Design review of the part built by this model. Coordinates are the model's own, in mm. A direction names the side the tool comes from. Give positions to 0.01 mm unless a question says otherwise; leave off trailing zeros. Order: outer loops, then holes, each group sorted by start corner. A loop starts at its lowest first (then second) coordinate and runs counter-clockwise, first axis right, second up. Notation, with made-up numbers: (63, 51.5) -> (92, 51.5) arc R29 cw to (92, 81.5) -> close; hole circle Ø6 at (30, -40). An arc over 180 degrees is marked (long way). One line per item, written item: value.
from build123d import *

# Parameters (mm, degrees)
SKETCH1_W           = 85
SKETCH1_H           = 115
SKETCH1_R           = 4.25
SKETCH1_R_2         = 8.5
SKETCH1_R_3         = 6.25
SKETCH1_R_4         = 2.5
SKETCH1_W_2         = 28
SKETCH1_H_2         = 17
BOSS_EXTRUDE1_DEPTH = 3
SKETCH2_W           = 88.917707464
SKETCH2_H           = 119.141928202
SKETCH2_W_2         = 85
SKETCH2_H_2         = 115
BOSS_EXTRUDE2_DEPTH = 50
SKETCH3_R           = 6
BOSS_EXTRUDE3_DEPTH = 50
SKETCH5_R           = 1.6
CUT_EXTRUDE1_DEPTH  = 30


with BuildPart() as part:
    # Sketch1 → Boss-Extrude1 (new body)
    with BuildSketch(Plane(origin=(0, 0, 0), x_dir=(1, 0, 0), z_dir=(0, 1, 0))):
        Rectangle(SKETCH1_W, SKETCH1_H)
        with Locations((-7.5, 47.5)):
            Circle(SKETCH1_R, mode=Mode.SUBTRACT)
        with Locations((-21, 21.25)):
            Circle(SKETCH1_R_2, mode=Mode.SUBTRACT)
        with Locations((6, 21.25)):
            Circle(SKETCH1_R_2, mode=Mode.SUBTRACT)
        with Locations((24.83030278, -21)):
            Circle(SKETCH1_R_3, mode=Mode.SUBTRACT)
        with Locations((24.83030278, -40)):
            Circle(SKETCH1_R_4, mode=Mode.SUBTRACT)
        with Locations((-7.5, -4.5)):
            Rectangle(SKETCH1_W_2, SKETCH1_H_2, mode=Mode.SUBTRACT)
    extrude(amount=BOSS_EXTRUDE1_DEPTH)

    # Sketch2 → Boss-Extrude2 (add)
    with BuildSketch(Plane(origin=(0, 3, 0), x_dir=(1, 0, 0), z_dir=(0, 1, 0))):
        Rectangle(SKETCH2_W, SKETCH2_H)
        Rectangle(SKETCH2_W_2, SKETCH2_H_2, mode=Mode.SUBTRACT)
    extrude(amount=-BOSS_EXTRUDE2_DEPTH)

    # Sketch3 → Boss-Extrude3 (add)
    with BuildSketch(Plane(origin=(0, 3, 0), x_dir=(1, 0, 0), z_dir=(0, 1, 0))):
        with Locations((44.458853732, 59.570964101)):
            Circle(SKETCH3_R)
        with Locations((-44.458853732, 59.570964101)):
            Circle(SKETCH3_R)
        with Locations((44.458853732, -59.570964101)):
            Circle(SKETCH3_R)
        with Locations((-44.458853732, -59.570964101)):
            Circle(SKETCH3_R)
    extrude(amount=-BOSS_EXTRUDE3_DEPTH)

    # Sketch5 → Cut-Extrude1 (cut)
    with BuildSketch(Plane.XZ.offset(47)):
        with Locations((-44.458853732, 59.570964101)):
            Circle(SKETCH5_R)
        with Locations((44.458853732, 59.570964101)):
            Circle(SKETCH5_R)
        with Locations((44.458853732, -59.570964101)):
            Circle(SKETCH5_R)
        with Locations((-44.458853732, -59.570964101)):
            Circle(SKETCH5_R)
    extrude(amount=-CUT_EXTRUDE1_DEPTH, mode=Mode.SUBTRACT)


solid = part.part
Item 1: Add section B-B on x = -7.5. Give the boundary of the cut face in (y, z).
Returned:
outline: (-47, -59.57) -> (3, -59.57) -> (3, -51.75) -> (0, -51.75) -> (0, -57.5) -> (-47, -57.5) -> close; (-47, 57.5) -> (0, 57.5) -> (0, 13) -> (3, 13) -> (3, 59.57) -> (-47, 59.57) -> close; (0, -43.25) -> (3, -43.25) -> (3, -4) -> (0, -4) -> close
Item 2: Add section D-D on y = -6.5. Give the boundary of the cut face in (x, z), plus the area to 3 significant figures.
Returned:
outline: (-44.46, -53.57) arc R6 ccw (long way) to (-38.46, -59.57) -> (38.46, -59.57) arc R6 ccw (long way) to (44.46, -53.57) -> (44.46, 53.57) arc R6 ccw (long way) to (38.46, 59.57) -> (-38.46, 59.57) arc R6 ccw (long way) to (-44.46, 53.57) -> close; hole (-42.5, -53.9) arc R6 cw to (-38.83, -57.5) -> (38.83, -57.5) arc R6 cw to (42.5, -53.9) -> (42.5, 53.9) arc R6 cw to (38.83, 57.5) -> (-38.83, 57.5) arc R6 cw to (-42.5, 53.9) -> close
area: 1,190 mm²
Item 3: Machinability: for faces 4 (the cylindrical face through (48.56, -21.65, 63.95)), 5 (the flat face through (44.459, -22, 1)), 6 (the flat face through (-44.459, -22, 1)), 7 (the flat face through (-44, -17, 60)), which of the approach directions +Z, -Z, +X, -X, +Y, -Y give a long, thin tool a straight path to every point of the face, cutting with its end or side? Answer none if there is none.
Returned:
face 4: +Y, -Y
face 5: +X, +Y, -Y
face 6: -X, +Y, -Y
face 7: -Y
Item 4: To check wall thickness, follow line 1 along Z through (x, y) = (-7.5, 2.3); line 2 along X through (y, z) = (1, -21); line 3 along X through (y, z) = (-30.5, -46). State the ranges of each line that lie inside material, in increasing order. Write a range as from..to.
Returned:
line 1: -59.57..-51.75, -43.25..-4, 13..59.57
line 2: -44.46..-29.5, -12.5..-2.5, 14.5..44.46
line 3: -44.46..-42.5, 42.5..44.46
Item 5: Clearance check with flat-ended pins moving along their axes: P1, Ø1, axis at y = -19, z = -13.5, coming from the +X side; P2, Ø1, axis at x = 44.5, z = -59.5, coming from the -Y side; P3, Ø3, axis at x = -38, y = -20.5, coming from the +Z side. State where each tip first meets the part, or that it passes through.
Returned:
P1: x = 44.46
P2: y = -17
P3: z = 62.95
Item 6: Add section C-C on z = -47.5. Give the boundary of the cut face in (x, y), plus the area to 3 significant figures.
Returned:
outline: (-44.46, -47) -> (-42.5, -47) -> (-42.5, 0) -> (-11.75, 0) -> (-11.75, 3) -> (-44.46, 3) -> close; (-3.25, 0) -> (42.5, 0) -> (42.5, -47) -> (44.46, -47) -> (44.46, 3) -> (-3.25, 3) -> close
area: 425 mm²
Item 7: Add section A-A on z = -21.25. Give the boundary of the cut face in (x, y), plus the area to 3 significant figures.
Returned:
outline: (-44.46, -47) -> (-42.5, -47) -> (-42.5, 0) -> (-29.5, 0) -> (-29.5, 3) -> (-44.46, 3) -> close; (-12.5, 0) -> (-2.5, 0) -> (-2.5, 3) -> (-12.5, 3) -> close; (14.5, 0) -> (42.5, 0) -> (42.5, -47) -> (44.46, -47) -> (44.46, 3) -> (14.5, 3) -> close
area: 349 mm²
Item 8: Draft analysis for pull direction Z (two halves, no side actions). For faces 1 (the cylindrical face through (-8.42, 1.48, -43.35)), 2 (the flat face through (0, -47, -59)), 3 (the flat face through (-1, -22, -59.571)), state which applies: pulls with the +Z half, pulls with the -Z half, needs draft (parallel to the pull), parting line crosses it, or undercut.
Returned:
face 1: undercut
face 2: needs draft
face 3: pulls with the -Z half
